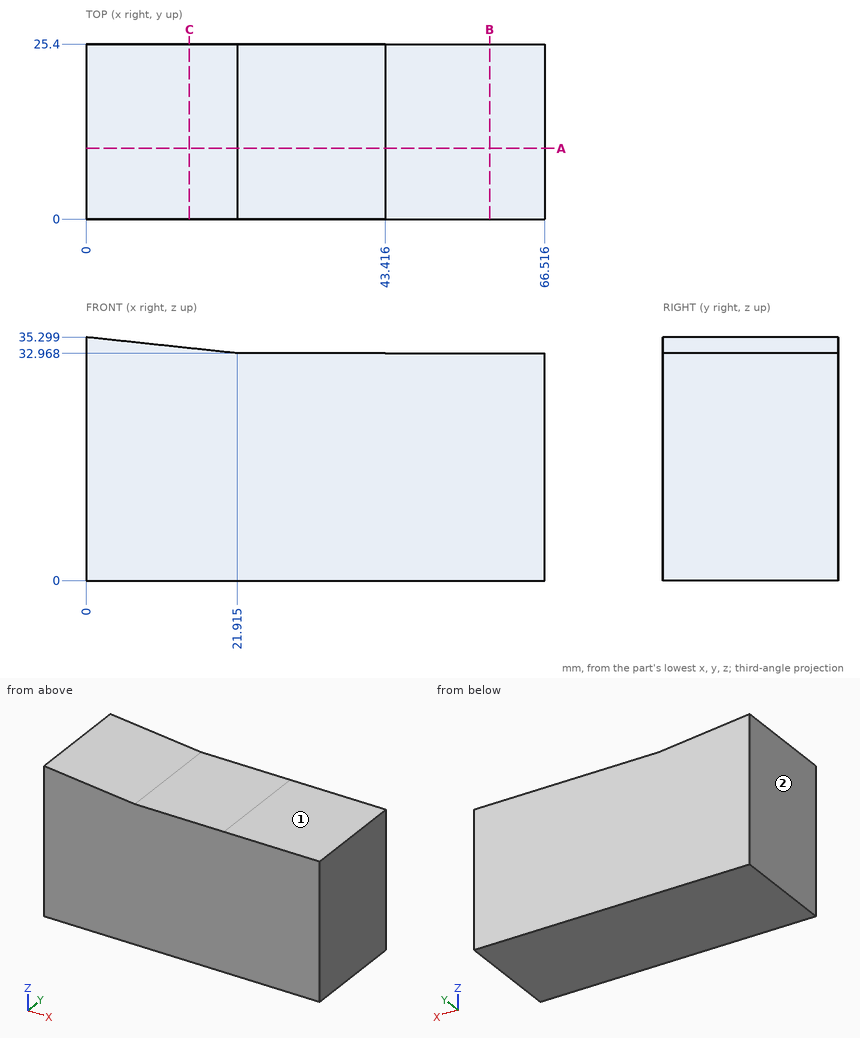
For this review, use the dimensioned drawing (mm, ordinates from the lowest corner) and the shaded views. A direction names the side the tool comes from. Give positions to 0.01 mm unless a question says otherwise; leave off trailing zeros. Loops run counter-clockwise (first coordinate to the right, second up) from the corner with the lowest first, then second, coordinate; pieces in that order, holes last.
Item 1: Tool access review of the marked faces 1 and 2: name each direction out of +Z, -Z, +X, -X, +Y, -Y from which nothing blocks a thin tool from reaching the whole face with its end or side.
Item 2: For line 1 along Z through (x, y) = (54, 15.75); line 2 along Z through (x, y) = (19, 9), list the stretches that pass through material, from the lowest coordinate up.
Item 3: Insertion check: pin 1 (7 mm diameter, centred on x = 57, y = 8, fed in from +Z). The pin has a flat end and moves straight along its axis. Give the tip position at first contact, or say it passes through.
Item 4: Take a section at A-A, the plane y = 10.25. State the section outline as (x, z) points (1 decimal).
Item 5: Take a section at C-C, the plane x = 15. State the section outline as (y, z) points, and give its area (3 significant figures).
Item 6: Take a section at B-B, the plane x = 58.5. State the section outline as (y, z) points, and give its area (3 significant figures).
Calculated:
1. face 1: +Z, +X, +Y, -Y
1. face 2: +Z, -Z, -X, +Y, -Y
2. line 1: z = 0 to 32.97
2. line 2: z = 0 to 33.28
3. pin 1: stops at z = 32.97
4. outline: (0, 0) - (66.5, 0) - (66.5, 33) - (21.9, 33) - (0, 35.3) - close
5. outline: (0, 0) - (25.4, 0) - (25.4, 33.7) - (0, 33.7) - close
5. area: 856 mm2
6. outline: (0, 0) - (25.4, 0) - (25.4, 32.97) - (0, 32.97) - close
6. area: 837 mm2
